Here's how the part is built. I have some questions about the finished solid (model axes, mm). Face numbers are marked on the shaded views. Coordinates: 2 decimals unless noted, no trailing zeros. Write each loop counter-clockwise with the first axis right and the second up, starting at its lowest first coordinate (ties: lowest second). Pieces come first, ordered by that corner, then holes. Notation, with made-up numbers: (-34, 62) -> (-21, 62) arc R31 ccw to (-21, 100) -> close; hole circle Ø3 at (-13.5, 77). An arc over 180 degrees is marked (long way). Use a Markdown table: item, result. Add a question column.
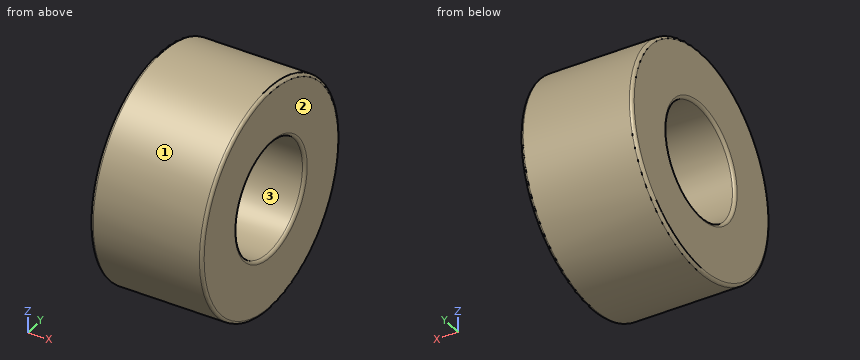
```python
from build123d import *

# Parameters (mm, degrees)
F0_R     = 19.05
F0_R_2   = 9.525
F1_DEPTH = 9.525
F2_R     = 0.5


with BuildPart() as f1:
    # F0 (on Right) → F1 (new body, symmetric)
    with BuildSketch(Plane.YZ):
        Circle(F0_R)
        Circle(F0_R_2, mode=Mode.SUBTRACT)
    extrude(amount=F1_DEPTH, both=True)

    # F2
    f2_edges = [f1.edges().sort_by_distance(p)[0] for p in [
        (9.525, -19.05, 0),
        (9.525, -9.525, 0),
        (-9.525, -19.05, 0),
        (-9.525, -9.525, 0),
    ]]
    fillet(f2_edges, radius=F2_R)


solid = f1.part
```
Q1. Suppose I cut it at A-A, the plane y = 0. Write out the boundary of the cut face in (x, z) (3 decimals), and give its area (3 significant figures).
Q2. Thinking about a two-plate mould opening in Y: for the marked faces 1, 2 and 3, which applies, released by +Y, released by -Y, zero draft, split by the parting line, or undercut?
Q3. Please list where these lines run through material, in increasing order: line 1 (Z direction, x = 4.5, y = 0) (3 decimals); line 2 (Y direction, x = -5.75, z = 2.5); line 3 (Z direction, x = 8, y = 6.5).
Q4. Will these pins go through, and if not, where does the flat tip stop? pin 1 (5 mm diameter, centred on x = -7, z = 7.5, fed in from -Y); pin 2 (2 mm diameter, centred on x = 0, y = -10, fed in from -Z); pin 3 (8 mm diameter, centred on x = -3.5, y = 13.5, fed in from -Z).
Q5. Suppose I cut it at C-C, the plane x = 4. Write out the boundary of the cut face in (y, z) (3 decimals).
Answer key:
| question | item | result |
|---|---|---|
| 1 | outline | (-9.525, -18.55) arc R0.5 ccw to (-9.025, -19.05) -> (9.025, -19.05) arc R0.5 ccw to (9.525, -18.55) -> (9.525, -10.025) arc R0.5 ccw to (9.025, -9.525) -> (-9.025, -9.525) arc R0.5 ccw to (-9.525, -10.025) -> close; (-9.525, 10.025) arc R0.5 ccw to (-9.025, 9.525) -> (9.025, 9.525) arc R0.5 ccw to (9.525, 10.025) -> (9.525, 18.55) arc R0.5 ccw to (9.025, 19.05) -> (-9.025, 19.05) arc R0.5 ccw to (-9.525, 18.55) -> close |
| 1 | area | 362 mm^2 |
| 2 | face 1 | split by the parting line |
| 2 | face 2 | zero draft |
| 2 | face 3 | undercut |
| 3 | line 1 | z = -19.05 to -9.525, 9.525 to 19.05 |
| 3 | line 2 | y = -18.89 to -9.19, 9.19 to 18.89 |
| 3 | line 3 | z = -17.91 to -6.96, 6.96 to 17.91 |
| 4 | pin 1 | stops at y = -18.38 |
| 4 | pin 2 | stops at z = -16.79 |
| 4 | pin 3 | stops at z = -16.51 |
| 5 | outline | circle Ø38.1 at (0, 0); hole circle Ø19.05 at (0, 0) |
